Check sheet for the modelled part. Datum: model origin and axes. Units: mm. A direction names the side the tool comes from. Round coordinates to 2 decimals unless told otherwise and drop trailing zeros. Order: outer loops, then holes, each group sorted by start corner. A loop starts at its lowest first (then second) coordinate and runs counter-clockwise, first axis right, second up.
(1) Tool access check on faces 4 (the cylindrical face through (12.669, 13.203, 2.535)), 5 (the flat face through (-29, 3.1, 2)). Record the directions out of +Z, -Z, +X, -X, +Y, -Y that give a thin tool (end or side, any length) a straight path to the whole face; none if there is none.
(2) Sectioned sample at B-B, the plane y = -11.2. Enter the section's corners in (x, z), and give its area (3 significant figures).
(3) Mould release check, pull along X, two halves, no side actions. Record for faces 1 (the flat face through (-59, 15.3, 2.5)), 2 (the cylindrical face through (11.218, -0.273, 2.535)), 3 (the flat face through (-21, 18.5, 2)): released by +X, released by -X, zero draft, split by the parting line, or undercut.
(4) Sectioned sample at D-D, the plane y = 12. Enter the section's corners in (x, z) (3 decimals).
(5) Sectioned sample at C-C, the plane x = -34.5. Enter the section's corners in (y, z), and give its area (3 significant figures).
(6) Thickness scan on probe 1 along Y at (x, z) = (-55.5, 3); probe 2 along Y at (x, z) = (13.3, 1.45); probe 3 along X at (y, z) = (11.2, 3.95). Record the ranges inside material, lowest first.
(7) Sectioned sample at A-A, the plane x = 13.3. Enter the section's corners in (y, z), and give its area (3 significant figures).
Autodesk Inventor part; units mm, degrees
ref_plane "YZ Plane" through (0, 0, 0) normal (1, 0, 0) x (0, 1, 0)
ref_plane "XZ Plane" through (0, 0, 0) normal (0, 1, 0) x (-1, 0, 0)
ref_plane "XY Plane" through (0, 0, 0) normal (0, 0, 1) x (1, 0, 0)
sketch "Sketch1" plane through (0, 0, 0) normal (0, 0, 1) x (1, 0, 0)
  line L0 (0, 0) -> (-60, 0) construction
  line L1 (0, 3.1) -> (-60, 3.1)
  line L2 (-60, -3.1) -> (0, -3.1)
  arc A0 (0, -3.1) -> (0, 3.1) centre (0, 0) ccw
  arc A1 (-60, 3.1) -> (-60, -3.1) centre (-60, 0) ccw
  line L3 (0, 11.2) -> (-60, 11.2) construction
  line L4 (0, 14.3) -> (-60, 14.3)
  line L5 (-60, 8.1) -> (0, 8.1)
  arc A2 (0, 8.1) -> (0, 14.3) centre (0, 11.2) ccw
  arc A3 (-60, 14.3) -> (-60, 8.1) centre (-60, 11.2) ccw
  line L6 (0, -11.2) -> (-60, -11.2) construction
  line L7 (0, -8.1) -> (-60, -8.1)
  line L8 (-60, -14.3) -> (0, -14.3)
  arc A4 (0, -14.3) -> (0, -8.1) centre (0, -11.2) ccw
  arc A5 (-60, -8.1) -> (-60, -14.3) centre (-60, -11.2) ccw
  line L9 (7.3, -3.9) -> (-7.3, -3.9) construction
  line L10 (-7.3, -3.9) -> (-7.3, -18.5) construction
  line L11 (-7.3, -18.5) -> (7.3, -18.5) construction
  line L12 (7.3, -18.5) -> (7.3, -3.9) construction
  line L13 (7.3, 3.9) -> (-7.3, 3.9) construction
  line L14 (-7.3, 3.9) -> (-7.3, 18.5) construction
  line L15 (-7.3, 18.5) -> (7.3, 18.5) construction
  line L16 (7.3, 18.5) -> (7.3, 3.9) construction
  line L17 (-7.3, -3.9) -> (7.3, -18.5) construction
  line L18 (7.3, -3.9) -> (-7.3, -18.5) construction
  line L19 (-7.3, 18.5) -> (7.3, 3.9) construction
  line L20 (7.3, 18.5) -> (-7.3, 3.9) construction
  line L21 (0, -25.9) -> (0, 25.9) construction
  line L22 (-60, 18.5) -> (7.3, 18.5)
  line L23 (7.3, 18.5) -> (7.3, -18.5)
  line L24 (7.3, -18.5) -> (-60, -18.5)
  line L25 (-60, -18.5) -> (-60, 18.5)
  line L26 (7.3, 18.5) -> (19.3, 18.5)
  line L27 (19.3, 18.5) -> (19.3, -18.5)
  line L28 (19.3, -18.5) -> (7.3, -18.5)
  line L29 (7.3, -18.5) -> (7.3, 18.5)
  point P0 (-30, 0)
  point P1 (-30, 11.2)
  point P2 (-30, -11.2)
  point P3 (0, -11.2)
  dimension "d0" = 6.2
  dimension "d1" = 14.6
  dimension "d2" = 14.6
  dimension "d5" = 60
  dimension "d11" = 11.2
  dimension "d12" = 5
  dimension "d13" = 5
  dimension "d17" = 37
  dimension "d18" = 12
extrude "Extrusion1" add sketch "Sketch1" along normal blind 5 contours L1 L25 L5 A2 L4 L22 L23 L24 L8 A4 L7 L2 A0 | L26 L27 L28 L23
chamfer "Chamfer1" distance 2 angle 45 6 edges at (-60, 14.3, 2.5) (-60, 8.1, 2.5) (-60, 3.1, 2.5) (-60, -3.1, 2.5) (-60, -8.1, 2.5) (-60, -14.3, 2.5)
sketch "Sketch3" plane through (0, 0, 0) normal (0, 0, -1) x (-1, 0, 0)
  line L0 (-19.3, 18.5) -> (-7.3, 18.5) construction
  line L1 (-7.3, 18.5) -> (-7.3, -18.5) construction
  line L2 (-7.3, -18.5) -> (-19.3, -18.5) construction
  line L3 (-19.3, -18.5) -> (-19.3, 18.5) construction
  line L4 (60, -18.5) -> (-19.3, -18.5) construction
  line L5 (-19.3, 18.5) -> (60, 18.5) construction
  line L6 (-13.3, 18.5) -> (-13.3, -18.5) construction
  line L7 (60, -18.5) -> (-19.3, -18.5) construction
  line L8 (75.86, 0) -> (-35.16, 0) construction
  point P0 (0, 0)
  point P1 (-13.3, 11.2)
  point P2 (-13.3, -11.2)
  point P3 (-13.3, 0)
  dimension "d19" = 12
  dimension "d20" = 6
  dimension "d21" = 22.4
  dimension "d22" = 37
hole "Hole1" at (13.3, 11.2, 0) at (13.3, -11.2, 0) at (13.3, 0, 0) direction (0, 0, 1) diameter 4.2 end through all
equation "\"d2\" = d1"
equation "\"d13\" = d12"
equation "\"d20\" = 0.5 * d19"
properties part number "SampleMountFingers" material "Aluminum 6061"
Derived:
1. face 4: +Z, -Z
1. face 5: +Z, -Z, -X
2. outline: (3.1, 0) - (11.2, 0) - (11.2, 5) - (3.1, 5) - close; (15.4, 0) - (19.3, 0) - (19.3, 5) - (15.4, 5) - close
2. area: 60.0 mm2
3. face 1: released by -X
3. face 2: undercut
3. face 3: zero draft
4. outline: (2.995, 0) - (11.358, 0) - (11.358, 5) - (2.995, 5) - close; (15.242, 0) - (19.3, 0) - (19.3, 5) - (15.242, 5) - close
5. outline: (-18.5, 0) - (-14.3, 0) - (-14.3, 5) - (-18.5, 5) - close; (-8.1, 0) - (-3.1, 0) - (-3.1, 5) - (-8.1, 5) - close; (3.1, 0) - (8.1, 0) - (8.1, 5) - (3.1, 5) - close; (14.3, 0) - (18.5, 0) - (18.5, 5) - (14.3, 5) - close
5. area: 92.0 mm2
6. probe 1: y = -18.5 to -14.3, -8.1 to -3.1, 3.1 to 8.1, 14.3 to 18.5
6. probe 2: y = -18.5 to -13.3, -9.1 to -2.1, 2.1 to 9.1, 13.3 to 18.5
6. probe 3: x = 3.1 to 11.2, 15.4 to 19.3
7. outline: (-18.5, 0) - (-13.3, 0) - (-13.3, 5) - (-18.5, 5) - close; (-9.1, 0) - (-2.1, 0) - (-2.1, 5) - (-9.1, 5) - close; (2.1, 0) - (9.1, 0) - (9.1, 5) - (2.1, 5) - close; (13.3, 0) - (18.5, 0) - (18.5, 5) - (13.3, 5) - close
7. area: 122 mm2
